Work out the finished part from the listing and answer in its coordinate system (mm). Give positions to 0.01 mm unless a question says otherwise; leave off trailing zeros. Write each loop counter-clockwise with the first axis right and the second up, starting at its lowest first coordinate (ties: lowest second). Pieces come first, ordered by that corner, then holes.
1) Given pin 1 Ø5 at (x, y) = (62, 4) entering from -Z; pin 2 Ø1.5 at (x, y) = (34, -4) entering from +Z; pin 3 Ø5 at (x, y) = (57, 3) entering from -Z, each flat-ended and moving along its own axis, determine where each tip first touches the part or whether it passes through.
2) Find section C-C (x = 72.5). Determine the outline of the cut face in (y, z).
3) Find section D-D (y = 3). Determine the outline of the cut face in (x, z).
4) Find section B-B (y = 0). Determine the outline of the cut face in (x, z), plus the area to 3 significant figures.
5) Straight lines are drawn through the part: probe 1 along X at (y, z) = (0, 2); probe 2 along Z at (x, y) = (60.5, 0); probe 3 along X at (y, z) = (-1.5, -4.5). For each, find the intervals that lie inside material, in ascending order.
6) Find section A-A (z = 0). Determine the outline of the cut face in (x, y), plus the area to 3 significant figures.
7) Determine the mould class of faces 1 (the face through (73.205, 0.225, 0.056)), 2 (the face through (27.99, -4.1, -1.3)), 3 (the face through (51.654, -1.532, -3.695)) for opening direction Y: pulls with the +Y half, pulls with the -Y half, needs draft (parallel to the pull), parting line crosses it, or undercut.
```python
from build123d import *

# Parameters (mm, degrees)
SKETCH1_R           = 12.5
BOSS_EXTRUDE1_DEPTH = 9
SKETCH2_R           = 8
BOSS_EXTRUDE2_DEPTH = 96
SKETCH4_R           = 1.5
CUT_EXTRUDE1_DEPTH  = 96
ESCALA1_SCALE       = 0.5


with BuildPart() as part:
    # Sketch1 → Boss-Extrude1 (new body)
    with BuildSketch(Plane(origin=(0, 0, 0), x_dir=(0, 0, -1), z_dir=(1, 0, 0))):
        Circle(SKETCH1_R)
    extrude(amount=BOSS_EXTRUDE1_DEPTH)

    # Sketch2 → Boss-Extrude2 (add)
    with BuildSketch(Plane(origin=(9, 0, 0), x_dir=(0, 0, -1), z_dir=(1, 0, 0))):
        Circle(SKETCH2_R)
    extrude(amount=BOSS_EXTRUDE2_DEPTH)

    # Sketch4 → Cut-Extrude1 (cut)
    with BuildSketch(Plane.XY.offset(8)):
        with Locations((98, 0)):
            Circle(SKETCH4_R)
    extrude(amount=-CUT_EXTRUDE1_DEPTH, mode=Mode.SUBTRACT)


with BuildPart() as part_1:
    # Escala1: scaled about (46.97958084, -3.1e-08, 3.35e-07)
    add(part.part.scale(ESCALA1_SCALE).moved(Location((23.48979042, -1.5e-08, 1.68e-07))))


solid = part_1.part
```
Results:
1. pin 1: stops at z = -3.71
1. pin 2: stops at z = 2.33
1. pin 3: stops at z = -3.97
2. outline: (-0.75, -3.93) - (-0.75, 3.93) arc R4 ccw to start; (0.75, -3.93) arc R4 ccw to (0.75, 3.93) - close
3. outline: (23.49, -5.48) - (27.99, -5.48) - (27.99, -2.65) - (75.99, -2.65) - (75.99, 2.65) - (27.99, 2.65) - (27.99, 5.48) - (23.49, 5.48) - close
4. outline: (23.49, -6.25) - (27.99, -6.25) - (27.99, -4) - (71.74, -4) - (71.74, 4) - (27.99, 4) - (27.99, 6.25) - (23.49, 6.25) - close; (73.24, -4) - (75.99, -4) - (75.99, 4) - (73.24, 4) - close
4. area: 428 mm2
5. probe 1: x = 23.49 to 71.74, 73.24 to 75.99
5. probe 2: z = -4 to 4
5. probe 3: x = 23.49 to 27.99
6. outline: (23.49, -6.25) - (27.99, -6.25) - (27.99, -4) - (75.99, -4) - (75.99, 4) - (27.99, 4) - (27.99, 6.25) - (23.49, 6.25) - close; hole circle Ø1.5 at (72.49, 0)
6. area: 438 mm2
7. face 1: undercut
7. face 2: needs draft
7. face 3: parting line crosses it
